Build history of the part. All positions in model axes, mm. A direction names the side the tool comes from. Round coordinates to 2 decimals unless told otherwise and drop trailing zeros. Write each loop counter-clockwise with the first axis right and the second up, starting at its lowest first coordinate (ties: lowest second). Pieces come first, ordered by that corner, then holes. Notation, with made-up numbers: (27.5, 39) -> (49.5, 39) arc R17 ccw to (49.5, 65) -> close; hole circle Ø11 at (11.5, 32.25). An arc over 180 degrees is marked (long way). Answer as CSV lines item,"result".
from build123d import *

# Parameters (mm, degrees)
SKETCH1_8_R         = 0.75
CUT_EXTRUDE3_DEPTH  = 3
SKETCH3_2_W         = 3
SKETCH3_2_H         = 3
BOSS_EXTRUDE3_DEPTH = 3
SKETCH5_R           = 0.75
BOSS_EXTRUDE4_DEPTH = 1


with BuildPart() as part:
    # Loft2: read off the stored shape, not the designer's step
    # Loft2: loft between two sections, ruled curve by curve
    loft2_from = [
        Edge.make_bspline([(1.060660172, -1.060660172, 0), (1.185660172, -0.935660172, 0), (1.297737894, -0.778019164, 0), (1.45548774, -0.413512879, 0), (1.5, -0.207106781, 0), (1.5, 0.207106781, 0), (1.45548774, 0.413512879, 0), (1.297737894, 0.778019164, 0), (1.185660172, 0.935660172, 0), (1.060660172, 1.060660172, 0)], [0, 0, 0, 0, 0.25, 0.25, 0.5, 0.5, 0.75, 0.75, 1, 1, 1, 1], 3),
        Edge.make_bspline([(1.060660172, 1.060660172, 0), (0.935660172, 1.185660172, 0), (0.778019164, 1.297737894, 0), (0.413512879, 1.45548774, 0), (0.207106781, 1.5, 0), (-0.207106781, 1.5, 0), (-0.413512879, 1.45548774, 0), (-0.778019164, 1.297737894, 0), (-0.935660172, 1.185660172, 0), (-1.060660172, 1.060660172, 0)], [0, 0, 0, 0, 0.25, 0.25, 0.5, 0.5, 0.75, 0.75, 1, 1, 1, 1], 3),
        Edge.make_bspline([(-1.060660172, -1.060660172, 0), (-0.935660172, -1.185660172, 0), (-0.778019164, -1.297737894, 0), (-0.413512879, -1.45548774, 0), (-0.207106781, -1.5, 0), (0.207106781, -1.5, 0), (0.413512879, -1.45548774, 0), (0.778019164, -1.297737894, 0), (0.935660172, -1.185660172, 0), (1.060660172, -1.060660172, 0)], [0, 0, 0, 0, 0.25, 0.25, 0.5, 0.5, 0.75, 0.75, 1, 1, 1, 1], 3),
        Edge.make_bspline([(-1.060660172, 1.060660172, 0), (-1.185660172, 0.935660172, 0), (-1.297737894, 0.778019164, 0), (-1.45548774, 0.413512879, 0), (-1.5, 0.207106781, 0), (-1.5, -0.207106781, 0), (-1.45548774, -0.413512879, 0), (-1.297737894, -0.778019164, 0), (-1.185660172, -0.935660172, 0), (-1.060660172, -1.060660172, 0)], [0, 0, 0, 0, 0.25, 0.25, 0.5, 0.5, 0.75, 0.75, 1, 1, 1, 1], 3),
    ]
    loft2_to = [
        Edge.make_bspline([(1.5, -1.5, 5), (1.5, -1.25, 5), (1.5, -1, 5), (1.5, -0.5, 5), (1.5, -0.25, 5), (1.5, 0.25, 5), (1.5, 0.5, 5), (1.5, 1, 5), (1.5, 1.25, 5), (1.5, 1.5, 5)], [0, 0, 0, 0, 0.25, 0.25, 0.5, 0.5, 0.75, 0.75, 1, 1, 1, 1], 3),
        Edge.make_bspline([(1.5, 1.5, 5), (1.25, 1.5, 5), (1, 1.5, 5), (0.5, 1.5, 5), (0.25, 1.5, 5), (-0.25, 1.5, 5), (-0.5, 1.5, 5), (-1, 1.5, 5), (-1.25, 1.5, 5), (-1.5, 1.5, 5)], [0, 0, 0, 0, 0.25, 0.25, 0.5, 0.5, 0.75, 0.75, 1, 1, 1, 1], 3),
        Edge.make_bspline([(-1.5, -1.5, 5), (-1.25, -1.5, 5), (-1, -1.5, 5), (-0.5, -1.5, 5), (-0.25, -1.5, 5), (0.25, -1.5, 5), (0.5, -1.5, 5), (1, -1.5, 5), (1.25, -1.5, 5), (1.5, -1.5, 5)], [0, 0, 0, 0, 0.25, 0.25, 0.5, 0.5, 0.75, 0.75, 1, 1, 1, 1], 3),
        Edge.make_bspline([(-1.5, 1.5, 5), (-1.5, 1.25, 5), (-1.5, 1, 5), (-1.5, 0.5, 5), (-1.5, 0.25, 5), (-1.5, -0.25, 5), (-1.5, -0.5, 5), (-1.5, -1, 5), (-1.5, -1.25, 5), (-1.5, -1.5, 5)], [0, 0, 0, 0, 0.25, 0.25, 0.5, 0.5, 0.75, 0.75, 1, 1, 1, 1], 3),
    ]
    loft2 = Solid(Shell([*[Face.make_surface_from_curves(loft2_from[k], loft2_to[k]) for k in range(4)], Face(Wire(loft2_from)), Face(Wire(loft2_to))]))
    add(loft2)

    # Sketch1<8> → Cut-Extrude3 (cut)
    with BuildSketch(Plane.XY):
        Circle(SKETCH1_8_R)
    extrude(amount=CUT_EXTRUDE3_DEPTH, mode=Mode.SUBTRACT)

    # Sketch3<2> → Boss-Extrude3 (add)
    with BuildSketch(Plane.XY.offset(5)):
        Rectangle(SKETCH3_2_W, SKETCH3_2_H)
    extrude(amount=BOSS_EXTRUDE3_DEPTH)

    # Sketch5 → Boss-Extrude4 (add)
    with BuildSketch(Plane(origin=(1.5, 0, 0), x_dir=(0, 0, -1), z_dir=(1, 0, 0))):
        with Locations(Location((-6.5, 0, 0), (0, 0, 270))):
            Circle(SKETCH5_R)
    extrude(amount=BOSS_EXTRUDE4_DEPTH)


solid = part.part
1. Cut at B-B, the plane x = 1.7. Write the cut outline in (y, z).
Results found:
outline,"circle Ø1.5 at (0, 6.5)"
2. Probe line 1 along Y through (x, z) = (0, 0.6); line 2 along Z through (x, y) = (-0.6, 0); line 3 along X through (y, z) = (-1.3, 6). List the from-to ranges inside material, lowest first.
Results found:
line 1,"y = -1.5 to -0.75, 0.75 to 1.5"
line 2,"z = 3 to 8"
line 3,"x = -1.5 to 1.5"
3. Cut at A-A, the plane z = 6.5. Write the cut outline in (x, y).
Results found:
outline,"(-1.5, -1.5) -> (1.5, -1.5) -> (1.5, -0.75) -> (2.5, -0.75) -> (2.5, 0.75) -> (1.5, 0.75) -> (1.5, 1.5) -> (-1.5, 1.5) -> close"
4. Which spindle directions (+Z, -Z, +X, -X, +Y, -Y) get a long thin tool onto all of the face, cutting with end or side? Do faces 1 (the cylindrical face through (1.993, -0.715, 6.275)), 2 (the flat face through (-1, 0, 0)), 3 (the flat face through (0, 0, 3)). Say none if no direction does.
Results found:
face 1,"+X"
face 2,"-Z, +X, -X, +Y, -Y"
face 3,"-Z"
